Part model, mm, in its own coordinate system. Coordinates: 2 decimals unless noted, no trailing zeros. Write each loop counter-clockwise with the first axis right and the second up, starting at its lowest first coordinate (ties: lowest second). Pieces come first, ordered by that corner, then holes. Notation, with made-up numbers: M 68,66 L 100,66 A19 cw 100,102 Z; hole C -17,79.25 d7. An arc over 180 degrees is marked long. Use a Markdown table: item, result. Add a question column.
Q1. Wall check: L1, parallel to Y at x = 64.5, z = 9.25; L2, parallel to Y at x = 169.5, z = 3.5; L3, parallel to X at y = 53, z = 9.75. Give the ranges that are in metal, low to high. Write a range as from..to.
Q2. Slice it at D-D on x = 167.5. Write the cut outline in (y, z).
Q3. Pin check, flat tips, straight feed: pin 1 Ø2 at (y, z) = (155, 6.5) entering from -X; pin 2 Ø3 at (x, z) = (100, 13) entering from +Y. Stop position of each tip, or through.
Q4. Slice it at C-C on y = 190.5. Write the cut outline in (x, z).
Q5. Slice it at A-A on x = 39. Write the cut outline in (y, z), then the cut area to 3 significant figures.
Q6. Slice it at B-B on z = 10.5. Write the cut outline in (x, y), then the cut area to 3 significant figures.
Q7. Mould opens along Y. For faces 1 (the cylindrical face through (29.25, 186.95, 8.88)), 2 (the flat face through (190.498, 367, 9)), 3 (the flat face through (150, 0, 9)) say: released by +Y, released by -Y, zero draft, split by the parting line, or undercut.
Autodesk Inventor part; units mm, degrees
ref_plane "YZ Plane" through (0, 0, 0) normal (1, 0, 0) x (0, 1, 0)
ref_plane "XZ Plane" through (0, 0, 0) normal (0, 1, 0) x (-1, 0, 0)
ref_plane "XY Plane" through (0, 0, 0) normal (0, 0, 1) x (1, 0, 0)
sketch "Sketch1" plane through (0, 0, 0) normal (0, 0, 1) x (1, 0, 0)
  circle A0 centre (190.5, 190.5) radius 161.29
  circle A1 centre (190.5, 190.5) radius 161.29
  line L0 (0, 269.4113) -> (111.5887, 381)
  line L1 (0, 269.4113) -> (157.8102, 269.4113) construction
  line L2 (0, 111.5878) -> (111.5895, 0)
  line L3 (269.4113, 0) -> (381, 111.5903)
  line L4 (380.9968, 269.4113) -> (269.4113, 381)
  line L5 (0, 0) -> (380.9968, 0)
  line L6 (380.9968, 0) -> (380.9968, 380.9968)
  line L7 (380.9968, 380.9968) -> (0, 380.9968)
  line L8 (0, 380.9968) -> (0, 0)
  line L9 (190.4984, 380.9968) -> (190.4984, 351.79)
  line L10 (190.4984, 29.21) -> (190.4984, 0)
  point P0 (111.5855, 380.9968)
  point P1 (111.5895, 0)
  point P2 (380.9968, 111.5871)
  point P3 (269.4145, 380.9968)
  dimension "d3" = 322.58
  dimension "d27" = 45
  dimension "d28" = 157.8102
  dimension "d30" = 157.8235
  dimension "d32" = 157.8218
  dimension "d40" = 157.808
  dimension "d42" = 380.9968
  dimension "d43" = 380.9968
  dimension "d44" = 190.5
  dimension "d45" = 190.5
  dimension "d46" = 111.5878
  dimension "d49" = 29.21
  dimension "d50" = 29.2068
  dimension "d51" = 269.4113
  dimension "d52" = 381
  dimension "d53" = 269.4113
  dimension "d54" = 157.821
  dimension "d55" = 111.5887
  dimension "d56" = 269.4113
  dimension "d57" = 111.5878
  dimension "d58" = 111.5895
  dimension "d59" = 111.5855
extrude "Extrusion3" add sketch "Sketch1" along normal blind 18.0086 contours A0 L10 L5 L2 L8 L0 L7 L9
properties part number "Tube Ring Half"
Recorded:
| question | item | result |
|---|---|---|
| 1 | L1 | 47.09..89.81, 291.19..333.91 |
| 1 | L2 | 0..30.58, 350.42..381 |
| 1 | L3 | 58.59..106.19 |
| 2 | outline | M 0,0 L 30.86,0 L 30.86,18.01 L 0,18.01 Z; M 350.14,0 L 381,0 L 381,18.01 L 350.14,18.01 Z |
| 3 | pin 1 | x = 0 |
| 3 | pin 2 | y = 370.91 |
| 4 | outline | M 0,0 L 29.21,0 L 29.21,18.01 L 0,18.01 Z |
| 5 | outline | M 72.59,0 L 135.16,0 L 135.16,18.01 L 72.59,18.01 Z; M 245.84,0 L 308.41,0 L 308.41,18.01 L 245.84,18.01 Z |
| 5 | area | 2,250 mm² |
| 6 | outline | M 0,111.59 L 111.59,0 L 190.5,0 L 190.5,29.21 A161.29 cw 190.5,351.79 L 190.5,381 L 111.59,381 L 0,269.41 Z |
| 6 | area | 19,300 mm² |
| 7 | face 1 | undercut |
| 7 | face 2 | zero draft |
| 7 | face 3 | released by -Y |
